Read the model definition and answer for the solid it produces. Units are mm, in the model's axes. A direction names the side the tool comes from. Give positions to 0.01 mm unless a question says otherwise; leave off trailing zeros. Write each loop counter-clockwise with the first axis right and the second up, starting at its lowest first coordinate (ties: lowest second). Pieces come first, ordered by that corner, then holes. Notation, with made-up numbers: (13, -30.75) -> (63, -30.75) arc R35 ccw to (63, 3.25) -> close; hole circle Ø8 at (16, -6). An arc over 180 degrees is marked (long way). Answer as CSV lines item,"result". Start each with the question number.
1. The part is cut by section C-C, the plane y = -16.5. Determine the outline of the cut face in (x, z), and give its area (3 significant figures).
2. The part is cut by section B-B, the plane x = 7.5. Determine the outline of the cut face in (y, z).
3. Find the intervals of material crossed by line 1 (Y direction, x = 18.5, z = 40); line 2 (Y direction, x = 33, z = 24.5); line 3 (Z direction, x = 10, y = -5), in increasing order.
4. Given pin 1 (6 mm diameter, centred on x = 15.5, z = 11, fed in from -Y); pin 2 (4 mm diameter, centred on x = 19, y = -15, fed in from -Z); pin 3 (3 mm diameter, centred on x = 39.5, y = 23, fed in from -Z), each flat-ended and moving along its own axis, determine where each tip first touches the part or whether it passes through.
5. For a pull along Z with two mould halves and no side action, classify faces 1 (the flat face through (26.62, -20.09, 74.42)), 2 (the flat face through (26.622, -21.546, -74.66)), 3 (the flat face through (54, 0, 0)), 4 (the flat face through (27, 0, 1.5)) as pulls with the +Z half, pulls with the -Z half, needs draft (parallel to the pull), parting line crosses it, or undercut.
6. The part is cut by section A-A, the plane z = 53.5. Determine the outline of the cut face in (x, y), and give its area (3 significant figures).
7. A tool of negligible diameter and unlimited length cuts with its end or side. For faces 5 (the flat face through (0, 0, 0)), 6 (the flat face through (26.622, 21.546, -74.66)), 7 (the flat face through (26.62, -22.57, 36.46)), 8 (the flat face through (26.622, 19.938, 35.734)), 9 (the flat face through (27, 23, -1)), from which of +Z, -Z, +X, -X, +Y, -Y can it reach the whole face along a straight path? Write none if from no direction.
from build123d import *

# Parameters (mm, degrees)
F1_DEPTH = 54


with BuildPart() as f1:
    # F0 (on Right) → F1 (new body)
    with BuildSketch(Plane.YZ):
        Polygon((-24, 0), (0, 0), (0, 1.5), (-18.518498, 1.5), (-21.397766, 70.939903), (-18.741725, 78.002092), (-19.159078, 78.27744), (-24, 70.939903), (-21.1, 1), (-24, 1), align=None)
    extrude(amount=F1_DEPTH)

    # F2: F1 across plane


with BuildPart() as f1_1:
    add(f1.part)
    add(f1.part.mirror(Plane.XZ))

    # F3: F1 across plane


with BuildPart() as f1_2:
    add(f1_1.part)
    add(f1_1.part.mirror(Plane.XY))


solid = f1_2.part
Results found:
1,outline,"(0, -1.5) -> (54, -1.5) -> (54, 1.5) -> (0, 1.5) -> close"
1,area,"162 mm²"
2,outline,"(-24, -70.94) -> (-19.16, -78.28) -> (-18.74, -78) -> (-21.4, -70.94) -> (-18.52, -1.5) -> (18.52, -1.5) -> (21.4, -70.94) -> (18.74, -78) -> (19.16, -78.28) -> (24, -70.94) -> (21.1, -1) -> (24, -1) -> (24, 1) -> (21.1, 1) -> (24, 70.94) -> (19.16, 78.28) -> (18.74, 78) -> (21.4, 70.94) -> (18.52, 1.5) -> (-18.52, 1.5) -> (-21.4, 70.94) -> (-18.74, 78) -> (-19.16, 78.28) -> (-24, 70.94) -> (-21.1, 1) -> (-24, 1) -> (-24, -1) -> (-21.1, -1) -> close"
3,line 1,"y = -22.72 to -20.11, 20.11 to 22.72"
3,line 2,"y = -22.07 to -19.47, 19.47 to 22.07"
3,line 3,"z = -1.5 to 1.5"
4,pin 1,"stops at y = -21.64"
4,pin 2,"stops at z = -1.5"
4,pin 3,"stops at z = -74.73"
5,face 1,"undercut"
5,face 2,"pulls with the -Z half"
5,face 3,"needs draft"
5,face 4,"pulls with the +Z half"
6,outline,"(0, -23.28) -> (54, -23.28) -> (54, -20.67) -> (0, -20.67) -> close; (0, 20.67) -> (54, 20.67) -> (54, 23.28) -> (0, 23.28) -> close"
6,area,"281 mm²"
7,face 5,"+Z, -Z, -X, +Y, -Y"
7,face 6,"-Z, +X, -X, +Y"
7,face 7,"+X, -X, -Y"
7,face 8,"+X, -X"
7,face 9,"+X, -X, +Y"
